CAD build for the part. Positions are in the model's coordinates, mm. A direction names the side the tool comes from. Coordinates: 2 decimals unless noted, no trailing zeros. Order: outer loops, then holes, each group sorted by start corner. A loop starts at its lowest first (then second) coordinate and runs counter-clockwise, first axis right, second up. Notation, with made-up numbers: (23.5, 82.25) - (46.5, 82.25) arc R9 ccw to (46.5, 99.25) - close; hole circle Ø10 at (86, -13.5). An arc over 180 degrees is marked (long way). Use one line per item in the form item = value.
```python
from build123d import *

# Parameters (mm, degrees)
PAD008_DEPTH    = 44
SKETCH009_W     = 9
SKETCH009_H     = 80
POCKET_DEPTH    = 15
SKETCH011_W     = 9
SKETCH011_H     = 80
POCKET001_DEPTH = 15
FILLET006_R     = 3


with BuildPart() as part:
    # Sketch007 → Pad008 (new body, symmetric)
    with BuildSketch(Plane.YZ):
        Polygon((122.8253676514, 151.0712742396), (139.8253676514, 151.0712742396), (139.8253676514, 174.0688329116), (131.9597393383, 195.6794690919), (115.9849647849, 189.8651266553), (122.8253676514, 171.0712742396), align=None)
    extrude(amount=PAD008_DEPTH, both=True)

    # Sketch009 (on Face4 of Pad008) → Pocket (cut)
    with BuildSketch(Plane(origin=(0, -47.4538119498, 130.378276799), x_dir=(0, -0.9396926208, -0.3420201433), z_dir=(0, -0.3420201433, 0.9396926208))):
        with Locations((-182.4279133617, 0)):
            Rectangle(SKETCH009_W, SKETCH009_H)
    extrude(amount=-POCKET_DEPTH, mode=Mode.SUBTRACT)

    # Sketch011 (on Face1 of Pocket) → Pocket001 (cut)
    with BuildSketch(Plane.YX.offset(-151.0712742396)):
        with Locations((131.3253676514, 0)):
            Rectangle(SKETCH011_W, SKETCH011_H)
    extrude(amount=-POCKET001_DEPTH, mode=Mode.SUBTRACT)

    # Fillet006
    fillet006_edges = [part.edges().sort_by_distance(p)[0] for p in [
        (0, 139.825368, 174.068833),
        (0, 122.825368, 171.071274),
        (0, 115.984965, 189.865127),
        (44, 123.972352, 192.772298),
        (0, 131.959739, 195.679469),
        (-44, 123.972352, 192.772298),
        (-44, 131.325368, 151.071274),
        (0, 122.825368, 151.071274),
        (0, 139.825368, 151.071274),
        (44, 131.325368, 151.071274),
        (-44, 135.892553, 184.874151),
        (-44, 139.825368, 162.570054),
        (-44, 119.405166, 180.4682),
        (-44, 122.825368, 161.071274),
        (44, 119.405166, 180.4682),
        (44, 122.825368, 161.071274),
        (44, 135.892553, 184.874151),
        (44, 139.825368, 162.570054),
    ]]
    fillet(fillet006_edges, radius=FILLET006_R)


with BuildPart() as part_1:
    # Body011 placement: moved
    add(part.part.moved(Location((0, -6, -3))))


solid = part_1.part
```
Item 1: Drop flat-ended pins along their axis: pin 1 (1 mm diameter, centred on x = 12.5, y = 126, fed in from +Z); pin 2 (10 mm diameter, centred on x = 12.5, y = 129.5, fed in from +Z); pin 3 (1.5 mm diameter, centred on x = 22.5, z = 171, fed in from -Y). Give the stop position or say it passes through.
Derived:
pin_1 = 191.52
pin_2 = 191.82
pin_3 = 115.49
Item 2: Cut at B-B, the plane x = -14.5. Write the cut outline in (y, z).
Derived:
outline = (111.01, 184.05) - (116.64, 168.57) arc R3 cw to (116.83, 167.54) - (116.83, 151.07) arc R3 ccw to (119.83, 148.07) - (120.83, 148.07) - (120.83, 163.07) - (129.83, 163.07) - (129.83, 148.07) - (130.83, 148.07) arc R3 ccw to (133.83, 151.07) - (133.83, 170.54) arc R3 ccw to (133.64, 171.57) - (126.99, 189.86) arc R3 ccw to (123.14, 191.65) - (122.2, 191.31) - (127.33, 177.22) - (118.87, 174.14) - (113.74, 188.23) - (112.8, 187.89) arc R3 ccw to start
Item 3: Cut at A-A, the plane z = 152.5. Write the cut outline in (x, y).
Derived:
outline = (-44, 119.83) arc R3 ccw to (-41, 116.83) - (41, 116.83) arc R3 ccw to (44, 119.83) - (44, 130.83) arc R3 ccw to (41, 133.83) - (-41, 133.83) arc R3 ccw to (-44, 130.83) - close; hole (-40, 120.83) - (40, 120.83) - (40, 129.83) - (-40, 129.83) - close
Item 4: Two-plate mould, pull along Y, no slides. Class faces 1 (the face through (-0.56, 124.73, 184.36)), 2 (the face through (43.14, 114.71, 176.51)), 3 (the face through (-43.145, 129.421, 180.533)), 4 (the face through (-1, 129.825, 155)): +Y half, -Y half, draft (parallel to the pull), parting line (faces both ways), or undercut.
Derived:
face_1 = undercut
face_2 = -Y half
face_3 = +Y half
face_4 = undercut
Item 5: 3-axis set-ups, long thin cutter, end or side, ignore diameter. For faces 5 (the face through (43.098, 117.681, 159.191)), 6 (the face through (0.56, 123.162, 175.698)), 7 (the face through (-43.145, 117.728, 159.191)), 8 (the face through (1, 116.825, 159)): which of +Z, -Z, +X, -X, +Y, -Y reach the whole face in a straight line?
Derived:
face_5 = -Z, +X, -Y
face_6 = none
face_7 = -Z, -X, -Y
face_8 = -Z, +X, -X, -Y
Item 6: Drill centre lines: line 1 (Y direction, x = 30, z = 155); line 2 (X direction, y = 121.75, z = 181); line 3 (X direction, y = 131, z = 153). Where is each one in solid material? Low to high. Write a range as [from, to].
Derived:
line_1 = [116.83, 120.83], [129.83, 133.83]
line_2 = [-44, -40], [40, 44]
line_3 = [-43.99, 43.99]
